The model under review builds one solid part; all positions refer to its coordinate system, in mm. Face numbers are marked on the shaded views. A direction names the side the tool comes from. Coordinates: 2 decimals unless noted, no trailing zeros. Write each loop counter-clockwise with the first axis right and the second up, starting at its lowest first coordinate (ties: lowest second). Pieces come first, ordered by that corner, then holes. Notation, with made-up numbers: (-34, -36.75) -> (-14, -36.75) arc R34 cw to (-14, 0.25) -> close; hole circle Ø8 at (13.25, -38). An arc over 180 degrees is marked (long way). Write each question's results on one line, items separated by ' | '.
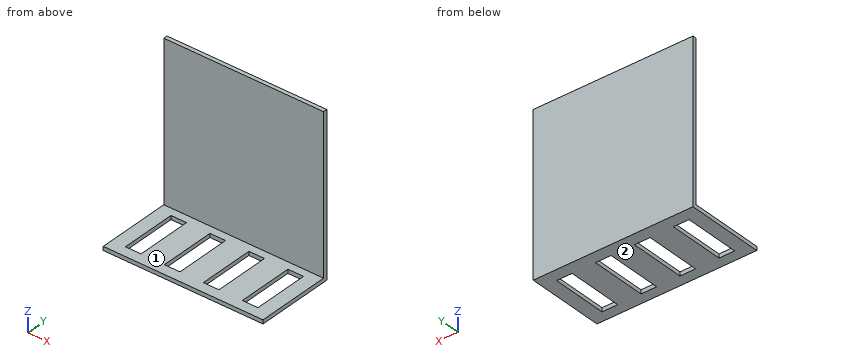
```python
from build123d import *

# Parameters (mm, degrees)
F1_E0_W  = 40
F1_E0_H  = 82
F2_DEPTH = 2
F1_E1_W  = 82
F1_E1_H  = 82
F3_DEPTH = 2
F4_W     = 8
F4_H     = 28.5714303715
F5_DEPTH = 2.001


with BuildPart() as f2:
    # F1_E0 (on explicit) → F2 (new body)
    with BuildSketch(Plane(origin=(0, -48.5075005184, 0), x_dir=(0, 1, 0), z_dir=(0, 0, -1))):
        with Locations((20, 41)):
            Rectangle(F1_E0_W, F1_E0_H)
    extrude(amount=-F2_DEPTH)

    # F1_E1 (on explicit) → F3 (join)
    with BuildSketch(Plane.ZX.offset(-8.5075005184)):
        with Locations((41, 41)):
            Rectangle(F1_E1_W, F1_E1_H)
    extrude(amount=-F3_DEPTH)

    # F4 (on face) → F5 (cut, through all)
    with BuildSketch(Plane.XY.offset(2)):
        with Locations((71, -28.857444413)):
            Rectangle(F4_W, F4_H)
        with Locations((51, -28.857444413)):
            Rectangle(F4_W, F4_H)
        with Locations((31, -28.857444413)):
            Rectangle(F4_W, F4_H)
        with Locations((11, -28.857444413)):
            Rectangle(F4_W, F4_H)
    extrude(amount=-F5_DEPTH, mode=Mode.SUBTRACT)


solid = f2.part
```
Q1. Add section B-B (y = -38.5). Write out the cut boundary in (x, z), plus the area to 3 significant figures.
Solution:
outline: (0, 0) -> (7, 0) -> (7, 2) -> (0, 2) -> close; (15, 0) -> (27, 0) -> (27, 2) -> (15, 2) -> close; (35, 0) -> (47, 0) -> (47, 2) -> (35, 2) -> close; (55, 0) -> (67, 0) -> (67, 2) -> (55, 2) -> close; (75, 0) -> (82, 0) -> (82, 2) -> (75, 2) -> close | area: 100 mm²
Q2. Machinability: for the marked faces 1 and 2, which of the approach directions +Z, -Z, +X, -X, +Y, -Y give a long, thin tool a straight path to every point of the face, cutting with its end or side? Answer none if there is none.
Solution:
face 1: +Z, +X, -X, -Y | face 2: -Z, +X, -X, +Y, -Y
Q3. Add section D-D (z = 30). Write out the cut boundary in (x, y), plus the area to 3 significant figures.
Solution:
outline: (0, -10.51) -> (82, -10.51) -> (82, -8.51) -> (0, -8.51) -> close | area: 164 mm²
Q4. For line 1 (Z direction, x = 59, y = -23); line 2 (Y direction, x = 71.5, z = 60), list the stretches that pass through material, from the lowest coordinate up. Write a range as from..to.
Solution:
line 1: 0..2 | line 2: -10.51..-8.51
Q5. Add section C-C (x = 44). Write out the cut boundary in (y, z).
Solution:
outline: (-48.51, 0) -> (-8.51, 0) -> (-8.51, 82) -> (-10.51, 82) -> (-10.51, 2) -> (-48.51, 2) -> close
Q6. Add section A-A (x = 28). Write out the cut boundary in (y, z).
Solution:
outline: (-48.51, 0) -> (-43.14, 0) -> (-43.14, 2) -> (-48.51, 2) -> close; (-14.57, 0) -> (-8.51, 0) -> (-8.51, 82) -> (-10.51, 82) -> (-10.51, 2) -> (-14.57, 2) -> close
Q7. Clearance check with a flat-ended pin moving along its axis: P1, Ø1, axis at x = 57.5, z = 62, coming from the -Y side. State where the tip first meets the part, or that it passes through.
Solution:
P1: y = -10.51
